Geometry: final body of the model. Coordinates: model frame, mm. Coordinates: 2 decimals unless noted, no trailing zeros. Write each loop counter-clockwise with the first axis right and the second up, starting at its lowest first coordinate (ties: lowest second). Pieces come first, ordered by that corner, then holes. Notation, with made-up numbers: (29.5, 35.5) - (82.5, 35.5) arc R24 ccw to (82.5, 52.5) - close; hole circle Ø10 at (34, 40). An arc over 180 degrees is marked (long way). Answer as a JSON object with one key per item and string values. Group by question number.
Item 1: Section A-A on x = 0. Return loops of the section in (y, z) (3 decimals), and give its area (3 significant figures).
Item 2: Line query: line 1 along X through (y, z) = (2.3, -3); line 2 along X through (y, z) = (2.3, -5); line 3 along Z through (x, y) = (-12, 1.1) (3 decimals). Output: solid intervals per line, ascending. Write a range as from..to.
Item 3: Section D-D on x = 14.5. Return loops of the section in (y, z) (3 decimals).
Item 4: Section B-B on z = 0. Return loops of the section in (x, y), and give its area (3 significant figures).
Item 5: Section C-C on y = 1.7. Return loops of the section in (x, z) (3 decimals).
```python
from build123d import *

# Parameters (mm, degrees)
SKETCH1_R           = 6.35
BOSS_EXTRUDE1_DEPTH = 2.54


with BuildPart() as part:
    # Sketch1 → Boss-Extrude1 (new body)
    with BuildSketch(Plane(origin=(0, 0, 0), x_dir=(1, 0, 0), z_dir=(0, 1, 0))):
        with BuildLine():
            Line((10.403230962, -7.284420742), (44.404903417, 41.275))
            Line((44.404903417, 41.275), (-44.404903417, 41.275))
            Line((-44.404903417, 41.275), (-10.403230962, -7.284420742))
            ThreePointArc((-10.403230962, -7.284420742), (0, -12.7), (10.403230962, -7.284420742))
        make_face()
        with Locations(Location((0, 0, 0), (0, 0, 270))):
            Circle(SKETCH1_R, mode=Mode.SUBTRACT)
    extrude(amount=BOSS_EXTRUDE1_DEPTH)


solid = part.part
```
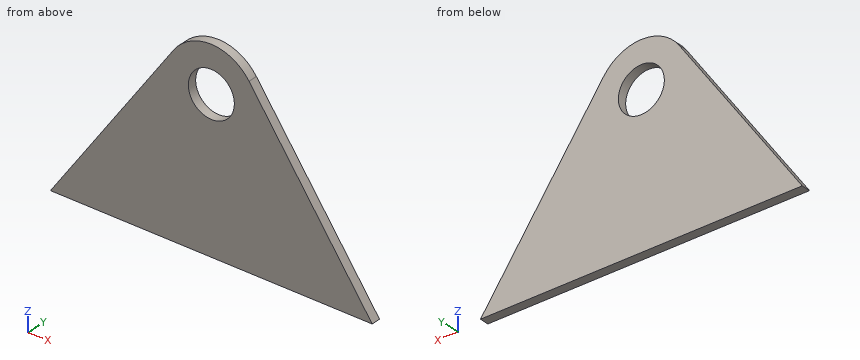
Checks:
{
 "1": {"outline": "(0, -41.275) - (2.54, -41.275) - (2.54, -6.35) - (0, -6.35) - close; (0, 6.35) - (2.54, 6.35) - (2.54, 12.7) - (0, 12.7) - close", "area": "105 mm^2"},
 "2": {"line 1": "-17.6..-5.6, 5.6..17.6", "line 2": "-19..-3.91, 3.91..19", "line 3": "-41.275..5.004"},
 "3": {"outline": "(0, -41.275) - (2.54, -41.275) - (2.54, 1.434) - (0, 1.434) - close"},
 "4": {"outline": "(-15.5, 0) - (-6.35, 0) - (-6.35, 2.54) - (-15.5, 2.54) - close; (6.35, 0) - (15.5, 0) - (15.5, 2.54) - (6.35, 2.54) - close", "area": "46.5 mm^2"},
 "5": {"outline": "(-44.405, -41.275) - (44.405, -41.275) - (10.403, 7.284) arc R12.7 ccw to (-10.403, 7.284) - close; hole circle Ø12.7 at (0, 0)"}
}
